Autodesk Inventor part; units mm, degrees
ref_plane "YZ Plane" through (0, 0, 0) normal (1, 0, 0) x (0, 1, 0)
ref_plane "XZ Plane" through (0, 0, 0) normal (0, 1, 0) x (-1, 0, 0)
ref_plane "XY Plane" through (0, 0, 0) normal (0, 0, 1) x (1, 0, 0)
sketch "Sketch1" plane through (0, 0, 0) normal (0, 0, 1) x (1, 0, 0)
  circle A0 centre (-35, 5) radius 2.5
  circle A1 centre (-35, -43.3013) radius 2.5
  circle A2 centre (-5, -43.3013) radius 2.5
  circle A3 centre (-5, 5) radius 2.5
  circle A4 centre (-5, 5) radius 3
  circle A5 centre (-35, 5) radius 3
  circle A6 centre (-5, -43.3013) radius 3
  circle A7 centre (-5, 5) radius 5
  line L0 (-5, 8) -> (-35, 8)
  line L1 (-5, 2) -> (-35, 2)
  circle A8 centre (-35, -43.3013) radius 5
  circle A9 centre (-5, -43.3013) radius 5
  circle A10 centre (-35, -43.3013) radius 3
  line L2 (-5, -40.3013) -> (-35, -40.3013)
  line L3 (-5, -46.3013) -> (-35, -46.3013)
  circle A11 centre (-35, 5) radius 5
  line L4 (-35, 8) -> (-39, 8)
  line L5 (-35, 2) -> (-39, 2)
  line L6 (-35, -40.3013) -> (-39, -40.3013)
  line L7 (-35, -46.3013) -> (-39, -46.3013)
  line L8 (-5, 10) -> (-35, 10)
  line L9 (-5, 0) -> (-35, 0)
  line L10 (-5, -38.3013) -> (-35, -38.3013)
  line L11 (-5, -48.3013) -> (-35, -48.3013)
  line L12 (-35, 0) -> (-35, -38.3013)
  line L13 (-39, 2) -> (-39, -40.3013)
  point P0 (0, 0)
  dimension "d0" = 6
  dimension "d1" = 6
  dimension "d3" = 6
  dimension "d4" = 10
  dimension "d5" = 10
  dimension "d6" = 6
  dimension "d7" = 10
extrude "Extrusion1" add sketch "Sketch1" along normal blind 6.5 contours A4 L0 A7 L1 | L0 A11 L8 A7 | A7 L9 A11 L1 | L0 L4 A11 | A11 L5 L1 | L12 A8 L13 A11 | A8 L2 L6 | L10 A9 L2 A8 | A9 L3 A6 L2 | L7 L3 A8 | A8 L3 A9 L11 picked at (-7.4012, 8.2796) picked at (-7.4012, -46.5809)
sketch "Sketch2" plane through (-35, -38.3013, 0) normal (1, 0, 0) x (0, 0, -1)
  line L0 (-6.5, 0) -> (-6.5, 38.3013)
  line L1 (-6.5, 38.3013) -> (-6.5, 40.3013)
  line L2 (-6.5, 38.3013) -> (-11.5, 38.3013)
  line L3 (-6.5, 38.3013) -> (-1.5, 38.3013) construction
  line L4 (-6.5, 0) -> (-11.5, 0)
  line L5 (-6.5, 40.3013) -> (-6.5, -2)
  line L6 (-6.5, 0) -> (-1.5, 0) construction
  line L7 (-11.5, 0) -> (-11.5, 38.3013)
  point P0 (0, 38.3013)
  dimension "d10" = 5
  dimension "d11" = 180
  dimension "d12" = 5
  dimension "d13" = 180
extrude "Extrusion2" add sketch "Sketch2" against normal blind 4
sketch "Sketch3" plane through (-35, -38.3013, 6.5) normal (0, -1, 0) x (1, 0, 0)
  line L0 (0, 5) -> (0, 0)
  line L1 (0, 5) -> (-4, 5)
  line L2 (-4, 0) -> (-4, 5)
  line L3 (0, 0) -> (-4, 0)
  line L4 (-4, 5) -> (-4, 4)
  line L5 (-4, 4) -> (0, 5)
  point P0 (35, -6.5)
  dimension "d16" = 1
extrude "Extrusion3" cut sketch "Sketch3" against normal up to surface (38.3013 mm away) contours L5 L2 L1
ref_plane "Work Plane1" through (-39, -18.1506, 10.5) normal (0.9701, 0, 0.2425) x (0, 1, 0)
sketch "Sketch5" plane through (-35, -38.3013, 0) normal (1, 0, 0) x (0, 0, -1)
  line L0 (0, 38.3013) -> (0, 48.3013)
  line L1 (0, 48.3013) -> (-6.5, 48.3013)
  line L2 (-6.5, 38.3013) -> (-6.5, 48.3013)
  line L3 (0, 38.3013) -> (-6.5, 38.3013)
  line L4 (0, -10) -> (0, 0)
  line L5 (0, 0) -> (-6.5, 0)
  line L6 (-6.5, -10) -> (-6.5, 0)
  line L7 (0, -10) -> (-6.5, -10)
  line L8 (0, 0) -> (0, 38.3013)
  line L9 (0, 38.3013) -> (-6.5, 38.3013)
  line L10 (-6.5, 38.3013) -> (-11.5, 38.3013)
  line L11 (-11.5, 38.3013) -> (-11.5, 0)
  line L12 (-11.5, 0) -> (-6.5, 0)
  line L13 (0, 0) -> (-6.5, 0)
  line L14 (0, 48.3013) -> (0, 50.3013)
  line L15 (0, 50.3013) -> (-17.5997, 50.3013)
  line L16 (0, -10) -> (0, -12)
  line L17 (0, -12) -> (-16.7586, -12)
  line L18 (-11.5, 0) -> (-11.5, -14.3259)
  line L19 (-6.5, 38.3013) -> (-11.5, 38.3013)
  line L20 (-11.5, 38.3013) -> (-11.5, 54.2478)
  line L21 (-6.5, 48.3013) -> (-17.5997, 48.3013)
  line L22 (-6.5, -8) -> (-6.5, -10)
  line L23 (-6.5, -10) -> (-16.7586, -10)
  line L24 (-6.5, 38.3013) -> (-6.5, 38.8013)
  line L25 (-6.5, 38.8013) -> (-12, 38.8013)
  line L26 (-6.5, 0) -> (-6.5, -2)
  line L27 (-6.5, 0) -> (-6.5, -0.5)
  line L28 (-6.5, -0.5) -> (-13.9811, -0.5)
  line L29 (-11.5, 38.3013) -> (-10.5, 38.3013)
  line L30 (-10.5, 38.3013) -> (-10.5, 53.5621)
  line L31 (-11.5, 38.3013) -> (-11.5, 0)
  line L32 (-11.5, 0) -> (-10.5, 0)
  line L33 (-10.5, 0) -> (-10.5, -14.7859)
  point P0 (0, 38.3013)
  point P1 (-10.5, -0.5)
  point P2 (-6.5, -0.5)
  point P3 (-11.5, -12)
  point P4 (-10.5, -10)
  point P5 (-11.5, 50.3013)
  point P6 (-10.5, 38.8013)
  point P7 (-10.5, 48.3013)
  dimension "d26" = 2
  dimension "d27" = 2
  dimension "d28" = 0.5
  dimension "d29" = 90
  dimension "d30" = 0.5
  dimension "d31" = 1
extrude "Extrusion5" add sketch "Sketch5" along normal blind 31 and the other way blind 4 contours L1 L21 L30 L15 L14 | L10 L30 L25 L2 | L10 L20 L25 L30 | L16 L17 L33 L23 L7 | L6 L28 L33 L12 | L30 L25 L20 L21 | L21 L20 L15 L30 | L33 L28 L18 L12 | L33 L17 L18 L23 | L23 L18 L28 L33
sketch "Sketch24" plane through (0, 0, 0) normal (0, 0, -1) x (-1, 0, 0)
  line L0 (39, 2) -> (39, -40.3013)
  line L1 (5, 2) -> (39, 2)
  arc A0 (5, 8) -> (5, 2) centre (5, 5) ccw
  line L2 (39, 8) -> (5, 8)
  arc A1 (39, 8) -> (35, 10) centre (35, 5) ccw
  line L3 (39, 10) -> (35, 10)
  line L4 (39, 12) -> (39, 10)
  line L5 (4, 12) -> (39, 12)
  line L6 (4, 10) -> (4, 12)
  line L7 (5, 10) -> (4, 10)
  arc A2 (5, 10) -> (5, 0) centre (5, 5) ccw
  line L8 (35, 0) -> (5, 0)
  line L9 (35, -38.3013) -> (35, 0)
  line L10 (5, -38.3013) -> (35, -38.3013)
  arc A3 (5, -38.3013) -> (5, -48.3013) centre (5, -43.3013) ccw
  line L11 (5, -48.3013) -> (4, -48.3013)
  line L12 (4, -50.3013) -> (4, -48.3013)
  line L13 (39, -50.3013) -> (4, -50.3013)
  line L14 (39, -48.3013) -> (39, -50.3013)
  line L15 (39, -48.3013) -> (35, -48.3013)
  arc A4 (35, -48.3013) -> (39, -46.3013) centre (35, -43.3013) ccw
  line L16 (5, -46.3013) -> (39, -46.3013)
  arc A5 (5, -40.3013) -> (5, -46.3013) centre (5, -43.3013) ccw
  line L17 (39, -40.3013) -> (5, -40.3013)
  line L18 (4, 12) -> (4, 0)
  arc A6 (4, 12) -> (0, 5) centre (8.7961, 4.6165) ccw
  arc A7 (0, -43.3013) -> (4, -50.3013) centre (6.6386, -44.1506) ccw
  line L19 (39, 8) -> (39, 12)
  line L20 (39, 0.5) -> (4, 0.5)
  line L21 (39, -46.3013) -> (39, -48.3982)
  line L22 (39, -48.3013) -> (39, -50.3013)
  point P0 (0, 0)
  point P1 (0.101, 6)
extrude "Extrusion23" add sketch "Sketch24" against normal blind 6.5 contours L18 L7 A2 | A2 A6 L6 L18 | L21 L15 A4 | A1 L3 L19 | A3 L11 L12 A7
sketch "Sketch25" plane through (-39, 2, 0) normal (-1, 0, 0) x (0, 0, 1)
  line L0 (6.5, -50.3013) -> (10.5, -50.3013)
  line L1 (10.5, -50.3013) -> (10.5, -40.8013)
  line L2 (10.5, -40.8013) -> (6.5, -40.8013)
  line L3 (6.5, -40.8013) -> (6.5, -50.3013)
  line L4 (0, -45.3013) -> (10.5, -45.3013)
  line L5 (6.5, -42.3013) -> (0, -42.3013)
  line L6 (0, 0) -> (0, -42.3013)
  point P0 (0, -2)
  point P1 (6.5, -45.3013)
extrude "Extrusion24" cut sketch "Sketch25" against normal blind 23.75
sketch "Sketch35" plane through (-39, -18.1506, 10.5) normal (0.9701, 0, 0.2425) x (0, 1, 0)
  line L0 (-20.1506, 0) -> (18.1506, 0)
  line L1 (0, 0) -> (0, 30)
  line L2 (0, 0) -> (30, 0) construction
  circle A0 centre (0, 14) radius 11
  line L3 (11, 14) -> (11, 0)
  line L4 (-11, 14) -> (-11, 0)
  line L5 (0, 25) -> (0, 35)
  point P0 (18.1506, -19.6454)
  point P1 (11, 0)
  dimension "d177" = 30
  dimension "d178" = 90
  dimension "d179" = 22
  dimension "d182" = 10
extrude "Extrusion34" add sketch "Sketch35" along normal blind 4
properties part number "CapTurnerV3"
Work out the finished part from the listing and answer in its coordinate system (mm). A direction names the side the tool comes from. Round coordinates to 2 decimals unless told otherwise and drop trailing zeros. Write each loop counter-clockwise with the first axis right and the second up, starting at its lowest first coordinate (ties: lowest second). Pieces come first, ordered by that corner, then holes. Notation, with made-up numbers: (1.25, 63) - (38.25, 63) arc R16 ccw to (38.25, 90) - close; hole circle Ø6 at (22, 69.5). An arc over 180 degrees is marked (long way). Return JSON: item names as keys, results as strings. Group by question number.
Q1. The part is cut by section B-B on y = 5. Write down the section's boundary in (x, z), then the cut area to 3 significant figures.
Q2. The mould has two halves that part along Z. Classify faces 5 (the flat face through (-15, -47, 6.5)), 6 (the flat face through (-37, -32, 11)), 7 (the flat face through (-22, -46.301, 3)), 8 (the flat face through (-42.074, -18.305, 22.797)): released by +Z, released by -Z, zero draft, split by the parting line, or undercut.
Q3. The part is cut by section D-D on y = -39.5. Write down the section's boundary in (x, z), then the cut area to 3 significant figures.
Q4. Find the intervals of material crossed by L1, parallel to Y at x = -8.5, z = 2.5; L2, parallel to Y at x = -28, z = 7; L3, parallel to Z at x = -7, y = 9, in increasing order.
Q5. The part is cut by section A-A on x = -30.5. Write down the section's boundary in (y, z), then the cut area to 3 significant figures.
Q6. For faces 1 (the cylindrical face through (-2, -43.2, 3.2)), 2 (the flat face through (-35, -19, 6)), 3 (the flat face through (-4, -46, 11)), 4 (the flat face through (-22, 5, 10.5)), determine the directions among +Z, -Z, +X, -X, +Y, -Y from which every point of the face is accessible in a straight line to the end or side of a thin tool.
Q7. Each of these flat-tipped pins is pushed along its axis until it touches: pin 1 Ø6 at (x, y) = (-24, 3) entering from +Z; pin 2 Ø6 at (x, z) = (-40, 21) entering from -Y; pin 3 Ø5 at (x, y) = (-6.5, -40.5) entering from -Z; pin 4 Ø12 at (y, z) = (-19, 15.5) entering from +X. Where does it stop, or does it pass through?
Q8. The part is cut by section C-C on y = -9. Write down the section's boundary in (x, z), then the cut area to 3 significant figures.
Solved:
{
 "1": {"outline": "(-39, 10.5) - (-4, 10.5) - (-4, 11.5) - (-39, 11.5) - close; (-2, 0) - (0, 0) - (0, 6.5) - (-2, 6.5) - close", "area": "48.0 mm²"},
 "2": {"face 5": "undercut", "face 6": "released by +Z", "face 7": "zero draft", "face 8": "released by -Z"},
 "3": {"outline": "(-39, 0) - (-1.75, 0) - (-1.75, 6.5) - (-39, 6.5) - close; (-39, 10.5) - (-4, 10.5) - (-4, 11.5) - (-39, 11.5) - close", "area": "277 mm²"},
 "4": {"L1": "-50.3 to -46.3, -40.3 to -38.3, 0 to 2, 8 to 12", "L2": "-50.3 to -48.3, -38.8 to -38.3, 0 to 0.5, 10 to 12", "L3": "0 to 6.5, 10.5 to 11.5"},
 "5": {"outline": "(-50.3, 0) - (-46.3, 0) - (-46.3, 6.5) - (-48.3, 6.5) - (-48.3, 10.5) - (-38.8, 10.5) - (-38.8, 6.5) - (-40.3, 6.5) - (-40.3, 0) - (-38.3, 0) - (-38.3, 11.5) - (-50.3, 11.5) - close; (0, 0) - (2, 0) - (2, 6.5) - (0.5, 6.5) - (0.5, 10.5) - (10, 10.5) - (10, 6.5) - (8, 6.5) - (8, 0) - (12, 0) - (12, 11.5) - (0, 11.5) - close", "area": "122 mm²"},
 "6": {"face 1": "-Z, -X", "face 2": "+Z, -Z, +X", "face 3": "+Z, +X, +Y, -Y", "face 4": "+X, -X"},
 "7": {"pin 1": "z = 11.5", "pin 2": "y = -29.15", "pin 3": "z = 0", "pin 4": "x = -35"},
 "8": {"outline": "(-43.88, 30) - (-39, 10.5) - (-39, 0) - (-35, 0) - (-35, 11.5) - (-35.12, 11.47) - (-40, 30.97) - close", "area": "124 mm²"}
}
